For this review, take the finished solid that the model builds, in its own axes (mm). A direction names the side the tool comes from. Round coordinates to 2 decimals unless told otherwise and drop trailing zeros. Order: outer loops, then holes, each group sorted by start corner. A loop starts at its lowest first (then second) coordinate and runs counter-clockwise, first axis right, second up. Notation, with made-up numbers: (-36, 85) -> (-8, 85) arc R21 ccw to (-8, 118) -> close; hole circle Ø4 at (-17, 15). An arc over 180 degrees is marked (long way). Use a Markdown table: item, result. Add a question column.
1) Consider section C-C (z = 10.5). State the section outline as (x, y) points, plus the area to 3 significant figures.
2) Consider section A-A (y = 0). State the section outline as (x, z) points, plus the area to 4 significant figures.
3) Clearance check with flat-ended pins moving along their axes: P1, Ø2, axis at y = 3, z = 9, coming from the -X side; P2, Ø2, axis at y = 2, z = 16.5, coming from the +X side; P3, Ø3, axis at x = 1.5, z = 11, coming from the +Y side. State where each tip first meets the part, or that it passes through.
4) Wall thickness on line 1 along Y through (x, z) = (0, 12.25); line 2 along Z through (x, y) = (3, -0.5); line 3 along Z through (x, y) = (-5, 2): over which ranges is each line inside the solid? List them lowest first. Write a range as [from, to].
5) Draft analysis for pull direction Z (two halves, no side actions). For faces 1 (the face through (1.5, 0.1, 8.5)), 2 (the face through (-1.08, -4.88, 18.49)), 3 (the face through (1, -1, 18)), 4 (the face through (1, 0, 7)), state which applies: pulls with the +Z half, pulls with the -Z half, needs draft (parallel to the pull), parting line crosses it, or undercut.
6) Machinability: for faces 5 (the face through (-0.27, -1.22, 13.18)), 6 (the face through (-0.75, 0.03, 12.92)), which of the approach directions +Z, -Z, +X, -X, +Y, -Y give a long, thin tool a straight path to every point of the face, cutting with its end or side? Answer none if there is none.
7) Consider section D-D (y = -3.5). State the section outline as (x, z) points, plus the area to 3 significant figures.
```python
from build123d import *

# Parameters (mm, degrees)
F1_R     = 7
F1_R_2   = 0.75
F2_DEPTH = 1.5
F3_R     = 1.25
F3_R_2   = 0.75
F4_DEPTH = 9.5
F5_R     = 5
F5_R_2   = 1.25
F5_R_3   = 0.75
F6_DEPTH = 1


with BuildPart() as f2:
    # F1 (on offset) → F2 (new body)
    with BuildSketch(Plane.XY.offset(7)):
        Circle(F1_R)
        Circle(F1_R_2, mode=Mode.SUBTRACT)
    extrude(amount=F2_DEPTH)

    # F3 (on face) → F4 (join)
    with BuildSketch(Plane.XY.offset(8.5)):
        Circle(F3_R)
        Circle(F3_R_2, mode=Mode.SUBTRACT)
    extrude(amount=F4_DEPTH)

    # F5 (on face) → F6 (join)
    with BuildSketch(Plane.XY.offset(18)):
        Circle(F5_R)
        Circle(F5_R_2, mode=Mode.SUBTRACT)
        Circle(F5_R_2)
        Circle(F5_R_3, mode=Mode.SUBTRACT)
    extrude(amount=F6_DEPTH)


solid = f2.part
```
Results list:
| question | item | result |
|---|---|---|
| 1 | outline | circle Ø2.5 at (0, 0); hole circle Ø1.5 at (0, 0) |
| 1 | area | 3.14 mm2 |
| 2 | outline | (-7, 7) -> (-0.75, 7) -> (-0.75, 19) -> (-5, 19) -> (-5, 18) -> (-1.25, 18) -> (-1.25, 8.5) -> (-7, 8.5) -> close; (0.75, 7) -> (7, 7) -> (7, 8.5) -> (1.25, 8.5) -> (1.25, 18) -> (5, 18) -> (5, 19) -> (0.75, 19) -> close |
| 2 | area | 36.75 mm2 |
| 3 | P1 | x = -6.67 |
| 3 | P2 | x = 0.75 |
| 3 | P3 | y = 1.25 |
| 4 | line 1 | [-1.25, -0.75], [0.75, 1.25] |
| 4 | line 2 | [7, 8.5], [18, 19] |
| 4 | line 3 | [7, 8.5] |
| 5 | face 1 | undercut |
| 5 | face 2 | needs draft |
| 5 | face 3 | undercut |
| 5 | face 4 | pulls with the -Z half |
| 6 | face 5 | none |
| 6 | face 6 | +Z, -Z |
| 7 | outline | (-6.06, 7) -> (6.06, 7) -> (6.06, 8.5) -> (-6.06, 8.5) -> close; (-3.57, 18) -> (3.57, 18) -> (3.57, 19) -> (-3.57, 19) -> close |
| 7 | area | 25.3 mm2 |
